Design review of the part built by this model. Coordinates are the model's own, in mm. Face numbers are marked on the shaded views. Round coordinates to 2 decimals unless told otherwise and drop trailing zeros. Loops run counter-clockwise (first coordinate to the right, second up) from the corner with the lowest first, then second, coordinate; pieces in that order, holes last. Notation, with made-up numbers: (53.25, 53) - (73.25, 53) arc R16 ccw to (73.25, 72) - close; hole circle Ø7 at (-35, 88.25). An arc over 180 degrees is marked (long way). Return JSON: item names as keys, results as strings. Group by question number.
from build123d import *

# Parameters (mm, degrees)
SCHIZZO1_W                   = 154
SCHIZZO1_H                   = 160
SCHIZZO1_R                   = 1.5
ESTRUSIONE_ESTRUSIONE1_DEPTH = 7
SCHIZZO2_R                   = 41
SCHIZZO2_R_2                 = 2.25
SCHIZZO2_W                   = 12
SCHIZZO2_H                   = 8
TAGLIO_ESTRUSIONE1_DEPTH     = 10
SCHIZZO3_R                   = 1.5
SCHIZZO3_W                   = 25
SCHIZZO3_H                   = 5
TAGLIO_ESTRUSIONE2_DEPTH     = 10
SCHIZZO5_W                   = 140
SCHIZZO5_H                   = 154
TAGLIO_ESTRUSIONE3_DEPTH     = 5
SCHIZZO6_R                   = 3
SCHIZZO6_R_2                 = 1.5
ESTRUSIONE_ESTRUSIONE2_DEPTH = 3
RACCORDO1_R                  = 2
SCHIZZO8_W                   = 154
SCHIZZO8_H                   = 7
TAGLIO_ESTRUSIONE4_DEPTH     = 0.5


with BuildPart() as part:
    # Schizzo1 → Estrusione-Estrusione1 (new body)
    with BuildSketch(Plane.XY):
        Rectangle(SCHIZZO1_W, SCHIZZO1_H)
        with Locations((-75, 65.34394728)):
            Circle(SCHIZZO1_R, mode=Mode.SUBTRACT)
        with Locations(Location((75, 65.34394728, 0), (0, 0, 180))):
            Circle(SCHIZZO1_R, mode=Mode.SUBTRACT)
        with Locations((75, -65.34394728)):
            Circle(SCHIZZO1_R, mode=Mode.SUBTRACT)
        with Locations(Location((-75, -65.34394728, 0), (0, 0, 180))):
            Circle(SCHIZZO1_R, mode=Mode.SUBTRACT)
    extrude(amount=ESTRUSIONE_ESTRUSIONE1_DEPTH)

    # Schizzo2 → Taglio-Estrusione1 (cut)
    with BuildSketch(Plane(origin=(0, 0, 0), x_dir=(-1, 0, 0), z_dir=(0, 0, -1))):
        with Locations((0, -38)):
            Circle(SCHIZZO2_R)
        with Locations((35.499999997, -2.500000003)):
            Circle(SCHIZZO2_R_2)
        with Locations(Location((35.499999997, -73.499999997, 0), (0, 0, 180))):
            Circle(SCHIZZO2_R_2)
        with Locations(Location((-35.499999997, -2.500000003, 0), (0, 0, 180))):
            Circle(SCHIZZO2_R_2)
        with Locations((-35.499999997, -73.499999997)):
            Circle(SCHIZZO2_R_2)
        with Locations((0, 10)):
            Rectangle(SCHIZZO2_W, SCHIZZO2_H)
    extrude(amount=-TAGLIO_ESTRUSIONE1_DEPTH, mode=Mode.SUBTRACT)

    # Schizzo3 → Taglio-Estrusione2 (cut)
    with BuildSketch(Plane(origin=(0, 0, 0), x_dir=(-1, 0, 0), z_dir=(0, 0, -1))):
        with Locations((17, 65)):
            Circle(SCHIZZO3_R)
        with Locations((17, 39)):
            Circle(SCHIZZO3_R)
        with Locations(Location((-17, 39, 0), (0, 0, 180))):
            Circle(SCHIZZO3_R)
        with Locations(Location((-17, 65, 0), (0, 0, 180))):
            Circle(SCHIZZO3_R)
        with Locations((0, 67.5)):
            Rectangle(SCHIZZO3_W, SCHIZZO3_H)
    extrude(amount=-TAGLIO_ESTRUSIONE2_DEPTH, mode=Mode.SUBTRACT)

    # Schizzo5 → Taglio-Estrusione3 (cut)
    with BuildSketch(Plane(origin=(0, 0, 0), x_dir=(-1, 0, 0), z_dir=(0, 0, -1))):
        Rectangle(SCHIZZO5_W, SCHIZZO5_H)
    extrude(amount=-TAGLIO_ESTRUSIONE3_DEPTH, mode=Mode.SUBTRACT)

    # Schizzo6 → Estrusione-Estrusione2 (add)
    # profile 1 of 2: a face of its own
    with BuildSketch(Plane(origin=(0, 0, 5), x_dir=(-1, 0, 0), z_dir=(0, 0, -1))):
        with Locations(Location((8, 37, 0), (0, 0, 180))):
            Circle(SCHIZZO6_R)
        with Locations((8, 37)):
            Circle(SCHIZZO6_R_2, mode=Mode.SUBTRACT)
    # profile 2 of 2: a face of its own
    with BuildSketch(Plane(origin=(0, 0, 5), x_dir=(-1, 0, 0), z_dir=(0, 0, -1))):
        with Locations(Location((-8, 37, 0), (0, 0, 180))):
            Circle(SCHIZZO6_R)
        with Locations(Location((-8, 37, 0), (0, 0, 180))):
            Circle(SCHIZZO6_R_2, mode=Mode.SUBTRACT)
    extrude(amount=ESTRUSIONE_ESTRUSIONE2_DEPTH)

    # Raccordo1
    raccordo1_edges = [part.edges().sort_by_distance(p)[0] for p in [
        (-11, 37, 5),
        (5, 37, 5),
    ]]
    fillet(raccordo1_edges, radius=RACCORDO1_R)

    # Schizzo8 → Taglio-Estrusione4 (cut)
    with BuildSketch(Plane(origin=(0, 80, 0), x_dir=(1, 0, 0), z_dir=(0, 1, 0))):
        with Locations((0, -3.5)):
            Rectangle(SCHIZZO8_W, SCHIZZO8_H)
    extrude(amount=-TAGLIO_ESTRUSIONE4_DEPTH, mode=Mode.SUBTRACT)


solid = part.part
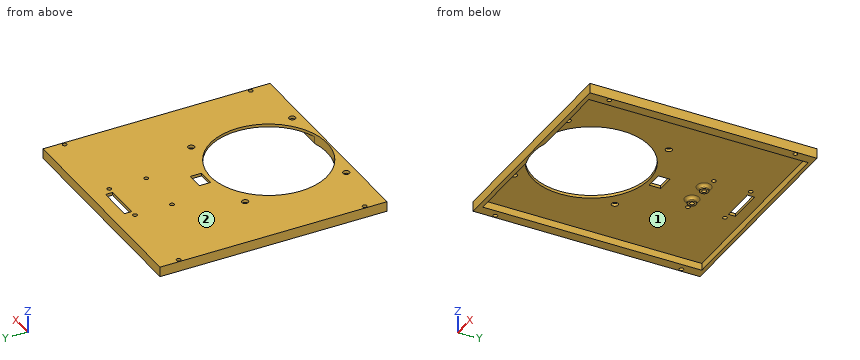
Q1. Add section B-B, the plane y = -38. State the section outline as (x, z) points, plus the area to 3 significant figures.
Q2. For line 1 (X direction, y = -53.5, z = 2.5); line 2 (X direction, y = -2.5, z = 6); line 3 (Y direction, x = 67, z = 4.25), list the stretches that pass through material, from the lowest coordinate up.
Q3. Add section D-D, the plane x = 59. State the section outline as (y, z) points, plus the area to 4 significant figures.
Q4. Add section A-A, the plane x = 0. State the section outline as (y, z) points.
Q5. Draft analysis for pull direction Y (two halves, no side actions). For the marked faces 1 and 2, state which applies: pulls with the +Y half, pulls with the -Y half, needs draft (parallel to the pull), parting line crosses it, or undercut.
Q6. Add section C-C, the plane x = 20.5. State the section outline as (y, z) points, plus the area to 3 significant figures.
Q7. Insertion check: pin 1 Ø6.5 at (x, y) = (-8.5, 37) entering from -Z; pin 2 Ø2.5 at (x, y) = (-75, -65.34) entering from +Z; pin 3 Ø3 at (x, y) = (58, 42.5) entering from -Z. Each pin has a flat end and moves straight along its axis. Give the tip position at first contact, or say it passes through.
Evaluation:
{
 "1": {"outline": "(-77, 0) - (-70, 0) - (-70, 5) - (-41, 5) - (-41, 7) - (-77, 7) - close; (41, 5) - (70, 5) - (70, 0) - (77, 0) - (77, 7) - (41, 7) - close", "area": "214 mm²"},
 "2": {"line 1": "-77 to -70, 70 to 77", "line 2": "-77 to -37.75, -33.25 to -20.51, 20.51 to 33.25, 37.75 to 77", "line 3": "-80 to -77, 77 to 79.5"},
 "3": {"outline": "(-80, 0) - (-77, 0) - (-77, 5) - (77, 5) - (77, 0) - (79.5, 0) - (79.5, 7) - (-80, 7) - close", "area": "346.5 mm²"},
 "4": {"outline": "(-80, 0) - (-79, 0) - (-79, 7) - (-80, 7) - close; (3, 5) - (6, 5) - (6, 7) - (3, 7) - close; (14, 5) - (65, 5) - (65, 7) - (14, 7) - close; (70, 5) - (77, 5) - (77, 0) - (79.5, 0) - (79.5, 7) - (70, 7) - close"},
 "5": {"face 1": "undercut", "face 2": "needs draft"},
 "6": {"outline": "(-80, 0) - (-77, 0) - (-77, 5) - (-73.51, 5) - (-73.51, 7) - (-80, 7) - close; (-2.49, 5) - (77, 5) - (77, 0) - (79.5, 0) - (79.5, 7) - (-2.49, 7) - close", "area": "204 mm²"},
 "7": {"pin 1": "z = 2", "pin 2": "through", "pin 3": "z = 5"}
}
